Autodesk Inventor part; units mm, degrees
ref_plane "YZ Plane" through (0, 0, 0) normal (1, 0, 0) x (0, 1, 0)
ref_plane "XZ Plane" through (0, 0, 0) normal (0, 1, 0) x (-1, 0, 0)
ref_plane "XY Plane" through (0, 0, 0) normal (0, 0, 1) x (1, 0, 0)
sketch "Esboço1" plane through (0, 0, 0) normal (0, 1, 0) x (-1, 0, 0)
  line L0 (-15, 25) -> (15, 25)
  line L1 (15, 25) -> (15, -25)
  line L2 (15, -25) -> (-15, -25)
  line L3 (-15, -25) -> (-15, 25)
  line L4 (-15, 25) -> (15, -25) construction
  line L5 (15, 25) -> (-15, -25) construction
  point P0 (0, 0)
  dimension "d0" = 30
  dimension "d1" = 50
extrude "Extrusão1" add sketch "Esboço1" along normal blind 70
sketch "Esboço2" plane through (15, 0, 25) normal (1, 0, 0) x (0, 0, -1)
  point P0 (25, 0)
sketch "Esboço3" plane through (15, 0, 25) normal (1, 0, 0) x (0, 0, -1)
  point P0 (25, 0)
sketch "Esboço4" plane through (15, 0, 25) normal (1, 0, 0) x (0, 0, -1)
  line L0 (0, 70) -> (20, 70)
  line L1 (20, 70) -> (20, 25)
  line L2 (20, 25) -> (0, 25)
  line L3 (0, 25) -> (0, 70)
  line L4 (50, 0) -> (50, 70)
  line L5 (0, 0) -> (50, 0)
  point P0 (25, 0)
  dimension "d4" = 30
  dimension "d5" = 25
extrude "Extrusão2" cut sketch "Esboço4" against normal blind 30
sketch "Esboço5" plane through (15, 0, 25) normal (1, 0, 0) x (0, 0, -1)
  point P0 (25, 0)
chamfer "Chanfro1" distance 15 angle 45 1 edges at (0, 70, 5) measured on face at (5, 70, -5)
Could you check a few things on this model? Use its own coordinates, in mm. A direction names the side the tool comes from. Round coordinates to 2 decimals unless told otherwise and drop trailing zeros. Order: outer loops, then holes, each group sorted by start corner. A loop starts at its lowest first (then second) coordinate and runs counter-clockwise, first axis right, second up.
(1) Imagine slicing it at B-B (z = 1). Write out the boundary of the cut face in (x, y), plus the area to 3 significant figures.
Response values:
outline: (-15, 0) - (15, 0) - (15, 59) - (-15, 59) - close
area: 1,770 mm2
(2) Imagine slicing it at C-C (y = 52.5). Write out the boundary of the cut face in (x, z), plus the area to 3 significant figures.
Response values:
outline: (-15, -25) - (15, -25) - (15, 5) - (-15, 5) - close
area: 900 mm2
(3) Which directions (+Z, -Z, +X, -X, +Y, -Y) give clear straight access to the entire face, cutting with the end or side of a thin tool? Please do faces 1 (the flat face through (0, 40, 5)), 2 (the flat face through (-15, 27, -5)).
Response values:
face 1: +Z, +X, -X, +Y
face 2: +Z, -Z, -X, +Y, -Y
(4) Please list where these lines run through material, in increasing order: line 1 along Z through (x, y) = (8.5, 44.5); line 2 along Y through (x, z) = (-1.75, 22.5); line 3 along Z through (x, y) = (4.25, 66).
Response values:
line 1: z = -25 to 5
line 2: y = 0 to 25
line 3: z = -25 to -6
(5) Imagine slicing it at A-A (x = 5). Write out the boundary of the cut face in (y, z), plus the area to 3 significant figures.
Response values:
outline: (0, -25) - (70, -25) - (70, -10) - (55, 5) - (25, 5) - (25, 25) - (0, 25) - close
area: 2,490 mm2
(6) I'm going to push flat-ended pins straight in: pin 1 (6 mm diameter, centred on x = 4.5, z = 14, fed in from -Y); pin 2 (15 mm diameter, centred on x = 0, y = 45.5, fed in from +Z); pin 3 (6 mm diameter, centred on x = 3.5, z = 16.5, fed in from +Y); pin 4 (1.5 mm diameter, centred on x = 2.5, z = 0.5, fed in from +Y). Where does each tip first touch, or does it pass through?
Response values:
pin 1: stops at y = 0
pin 2: stops at z = 5
pin 3: stops at y = 25
pin 4: stops at y = 60.25
